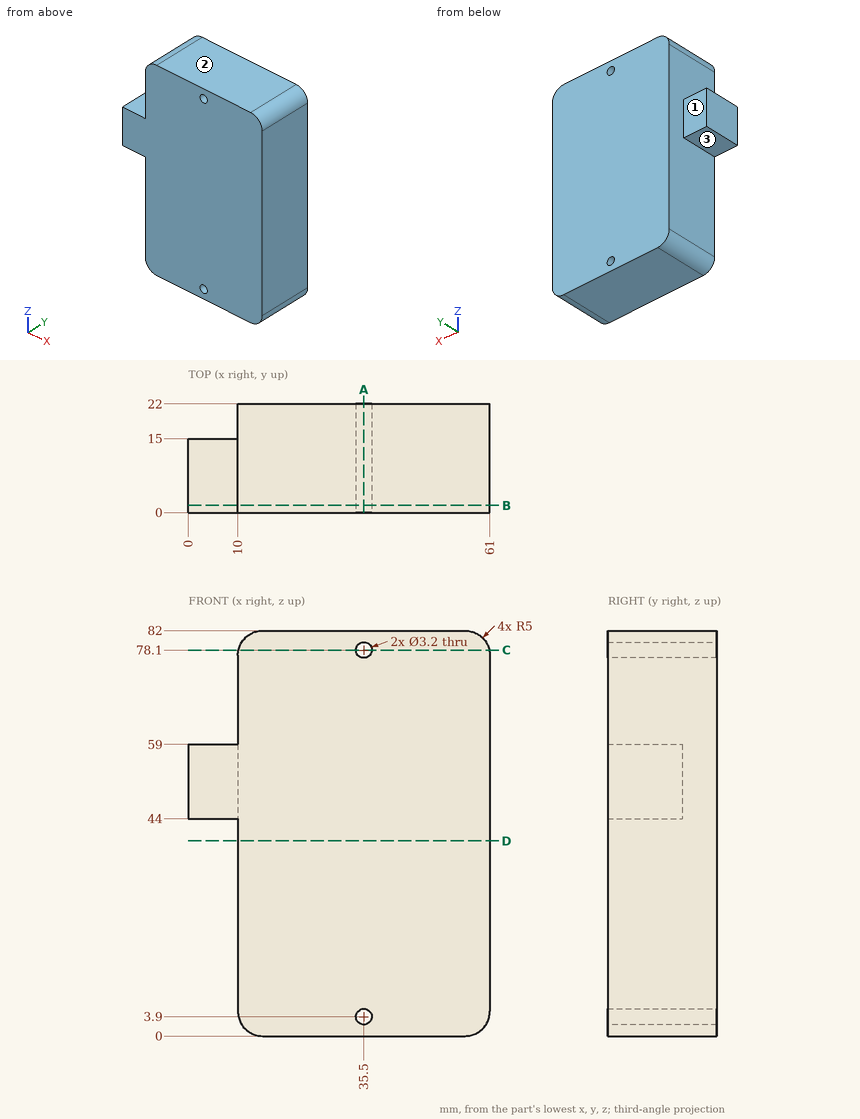
Part print with two shaded views. Sizes in mm from the minimum x, y, z corner. A direction names the side the tool comes from. Coordinates: 2 decimals unless noted, no trailing zeros. Loops run counter-clockwise (first coordinate to the right, second up) from the corner with the lowest first, then second, coordinate; pieces in that order, holes last. Notation, with made-up numbers: (51.25, 69.25) -> (66.25, 69.25) arc R30 cw to (66.25, 93.25) -> close; hole circle Ø6 at (-40, 22.25). An arc over 180 degrees is marked (long way). Answer as a JSON object with one key per item and string values.
Q1. Cut at D-D (z = 39.5). List the corners of the cut face in (x, y).
Report:
{"outline": "(10, 0) -> (61, 0) -> (61, 22) -> (10, 22) -> close"}
Q2. 3-axis set-ups, long thin cutter, end or side, ignore diameter. For the marked faces 1, 2 and 3: which of +Z, -Z, +X, -X, +Y, -Y reach the whole face in a straight line?
Report:
{"face 1": "+Z, -Z, -X, +Y", "face 2": "+Z, +X, -X, +Y, -Y", "face 3": "-Z, -X, +Y, -Y"}
Q3. Probe probe 1 along X at (y, z) = (2, 23); probe 2 along X at (y, z) = (13, 78.1); probe 3 along Z at (x, y) = (12, 19). List the from-to ranges inside material, lowest first.
Report:
{"probe 1": "x = 10 to 61", "probe 2": "x = 10.12 to 33.9, 37.1 to 60.88", "probe 3": "z = 1 to 81"}
Q4. Cut at C-C (z = 78.1). List the corners of the cut face in (x, y).
Report:
{"outline": "(10.12, 0) -> (33.9, 0) -> (33.9, 22) -> (10.12, 22) -> close; (37.1, 0) -> (60.88, 0) -> (60.88, 22) -> (37.1, 22) -> close"}
Q5. Cut at B-B (y = 1.5). List the corners of the cut face in (x, z).
Report:
{"outline": "(0, 44) -> (10, 44) -> (10, 5) arc R5 ccw to (15, 0) -> (56, 0) arc R5 ccw to (61, 5) -> (61, 77) arc R5 ccw to (56, 82) -> (15, 82) arc R5 ccw to (10, 77) -> (10, 59) -> (0, 59) -> close; hole circle Ø3.2 at (35.5, 3.9); hole circle Ø3.2 at (35.5, 78.1)"}
Q6. Cut at A-A (x = 35.5). List the corners of the cut face in (y, z).
Report:
{"outline": "(0, 0) -> (22, 0) -> (22, 2.3) -> (0, 2.3) -> close; (0, 5.5) -> (22, 5.5) -> (22, 76.5) -> (0, 76.5) -> close; (0, 79.7) -> (22, 79.7) -> (22, 82) -> (0, 82) -> close"}
Q7. Flat gauge pins, fed straight in: P1, Ø3, axis at x = 2.5, y = 5, coming from the +Z side; P2, Ø1.5, axis at y = 4.5, z = 23.5, coming from the -X side; P3, Ø5, axis at x = 3.5, z = 53, coming from the +Y side. Where does each tip first touch, or does it go through?
Report:
{"P1": "stops at z = 59", "P2": "stops at x = 10", "P3": "stops at y = 15"}
